For this review, use the dimensioned drawing (mm, ordinates from the lowest corner) and the shaded views. Coordinates: 2 decimals unless noted, no trailing zeros. Order: outer loops, then holes, each group sorted by start corner. A loop starts at its lowest first (then second) coordinate and runs counter-clockwise, first axis right, second up. Notation, with made-up numbers: (-12.5, -8.75) -> (23.5, -8.75) arc R18 ccw to (23.5, 15.25) -> close; hole circle Ø10 at (14.25, 11.25). An arc over 180 degrees is marked (long way). Use one line per item in the form item = value. Start each with the question number.
(1) Take a section at B-B (y = 2.75). State the section outline as (x, z) points.
(2) Insertion check: pin 1 Ø3 at (x, z) = (30, 10) entering from +Y; pin 2 Ø6 at (x, z) = (10, 10) entering from +Y. Each pin has a flat end and moves straight along its axis. Give the tip position at first contact, or say it passes through.
(3) Take a section at A-A (x = 190). State the section outline as (y, z) points, then the cut area to 3 significant figures.
(4) Wall thickness on line 1 along X through (y, z) = (4.75, 10); line 2 along Z through (x, y) = (90, 4.75); line 3 along X through (y, z) = (2.5, 7.5): over which ranges is each line inside the solid? List them lowest first.
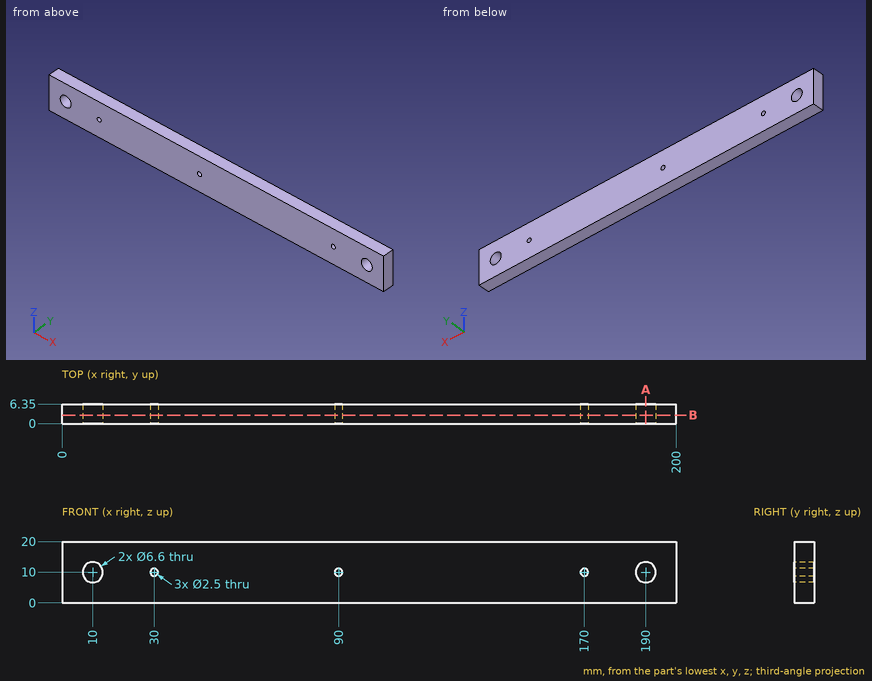
Findings:
q1.outline = (0, 0) -> (200, 0) -> (200, 20) -> (0, 20) -> close; hole circle Ø6.6 at (10, 10); hole circle Ø2.5 at (30, 10); hole circle Ø2.5 at (90, 10); hole circle Ø2.5 at (170, 10); hole circle Ø6.6 at (190, 10)
q2.pin_1 = 6.35
q2.pin_2 = through
q3.outline = (0, 0) -> (6.35, 0) -> (6.35, 6.7) -> (0, 6.7) -> close; (0, 13.3) -> (6.35, 13.3) -> (6.35, 20) -> (0, 20) -> close
q3.area = 85.1 mm²
q4.line_1 = 0 to 6.7, 13.3 to 28.75, 31.25 to 88.75, 91.25 to 168.75, 171.25 to 186.7, 193.3 to 200
q4.line_2 = 0 to 8.75, 11.25 to 20
q4.line_3 = 0 to 7.85, 12.15 to 187.85, 192.15 to 200
